from build123d import *

# Parameters (mm, degrees)
F0_W      = 88.9
F0_H      = 228.6
F1_DEPTH  = 19.05
F3_DEPTH  = 19.051
F4_R      = 4.7625
F5_DEPTH  = 5
F6_R      = 2.1
F7_DEPTH  = 12.7
F8_R      = 2.1
F9_DEPTH  = 12.7
F10_R     = 2.1
F10_R_2   = 2.0955
F11_DEPTH = 12.7
F12_W     = 37.5
F12_H     = 142.00124
F13_DEPTH = 0.889
F14_R     = 3.175
F15_DEPTH = 19.051


with BuildPart() as f1:
    # F0 (on Front) → F1 (new body)
    with BuildSketch(Plane.XZ):
        Rectangle(F0_W, F0_H)
    extrude(amount=-F1_DEPTH)

    # F2 (on face) → F3 (cut, through all)
    with BuildSketch(Plane.XZ):
        with BuildLine():
            ThreePointArc((-12.5, 90.3), (-15, 92.8), (-17.5, 90.3))
            Line((-17.5, 90.3), (-12.5, 90.3))
        make_face()
        with BuildLine():
            ThreePointArc((17.5, 90.3), (15, 92.8), (12.5, 90.3))
            Line((12.5, 90.3), (17.5, 90.3))
        make_face()
        with BuildLine():
            Line((17.5, 90.3), (12.5, 90.3))
            ThreePointArc((12.5, 90.3), (15, 87.8), (17.5, 90.3))
        make_face()
        with BuildLine():
            Line((-12.5, 90.3), (-17.5, 90.3))
            ThreePointArc((-17.5, 90.3), (-15, 87.8), (-12.5, 90.3))
        make_face()
        with BuildLine():
            ThreePointArc((-12.5, 60.3), (-15, 62.8), (-17.5, 60.3))
            Line((-17.5, 60.3), (-12.5, 60.3))
        make_face()
        with BuildLine():
            ThreePointArc((17.5, 60.3), (15, 62.8), (12.5, 60.3))
            Line((12.5, 60.3), (17.5, 60.3))
        make_face()
        with BuildLine():
            Line((17.5, 60.3), (12.5, 60.3))
            ThreePointArc((12.5, 60.3), (15, 57.8), (17.5, 60.3))
        make_face()
        with BuildLine():
            Line((-12.5, 60.3), (-17.5, 60.3))
            ThreePointArc((-17.5, 60.3), (-15, 57.8), (-12.5, 60.3))
        make_face()
        with BuildLine():
            ThreePointArc((-12.5, 15.3), (-15, 17.8), (-17.5, 15.3))
            Line((-17.5, 15.3), (-12.5, 15.3))
        make_face()
        with BuildLine():
            ThreePointArc((17.5, 15.3), (15, 17.8), (12.5, 15.3))
            Line((12.5, 15.3), (17.5, 15.3))
        make_face()
        with BuildLine():
            Line((17.5, 15.3), (12.5, 15.3))
            ThreePointArc((12.5, 15.3), (15, 12.8), (17.5, 15.3))
        make_face()
        with BuildLine():
            Line((-12.5, 15.3), (-17.5, 15.3))
            ThreePointArc((-17.5, 15.3), (-15, 12.8), (-12.5, 15.3))
        make_face()
        with BuildLine():
            ThreePointArc((-12.5, -14.7), (-15, -12.2), (-17.5, -14.7))
            Line((-17.5, -14.7), (-12.5, -14.7))
        make_face()
        with BuildLine():
            ThreePointArc((17.5, -14.7), (15, -12.2), (12.5, -14.7))
            Line((12.5, -14.7), (17.5, -14.7))
        make_face()
        with BuildLine():
            Line((17.5, -14.7), (12.5, -14.7))
            ThreePointArc((12.5, -14.7), (15, -17.2), (17.5, -14.7))
        make_face()
        with BuildLine():
            Line((-12.5, -14.7), (-17.5, -14.7))
            ThreePointArc((-17.5, -14.7), (-15, -17.2), (-12.5, -14.7))
        make_face()
    extrude(amount=-F3_DEPTH, mode=Mode.SUBTRACT)

    # F4 (on face) → F5 (cut)
    with BuildSketch(Plane.XZ):
        with Locations((-15, -14.7)):
            Circle(F4_R)
        with Locations((15, -14.7)):
            Circle(F4_R)
        with Locations((15, 15.3)):
            Circle(F4_R)
        with Locations((-15, 15.3)):
            Circle(F4_R)
        with Locations((-15, 60.3)):
            Circle(F4_R)
        with Locations((15, 60.3)):
            Circle(F4_R)
        with Locations((-15, 90.3)):
            Circle(F4_R)
        with Locations((15, 90.3)):
            Circle(F4_R)
    extrude(amount=-F5_DEPTH, mode=Mode.SUBTRACT)

    # F6 (on face) → F7 (cut)
    with BuildSketch(Plane(origin=(-44.45, 0, 0), x_dir=(0, -1, 0), z_dir=(-1, 0, 0))):
        with Locations((-9.525, 88.9)):
            Circle(F6_R)
        with Locations((-9.525, 63.5)):
            Circle(F6_R)
        with Locations((-9.525, 38.1)):
            Circle(F6_R)
        with Locations((-9.525, 12.7)):
            Circle(F6_R)
        with Locations((-9.525, -12.7)):
            Circle(F6_R)
        with Locations((-9.525, -38.1)):
            Circle(F6_R)
        with Locations((-9.525, -63.5)):
            Circle(F6_R)
        with Locations((-9.525, -88.9)):
            Circle(F6_R)
    extrude(amount=-F7_DEPTH, mode=Mode.SUBTRACT)

    # F8 (on face) → F9 (cut)
    with BuildSketch(Plane.YZ.offset(44.45)):
        with Locations((9.525, 88.9)):
            Circle(F8_R)
        with Locations((9.525, 63.5)):
            Circle(F8_R)
        with Locations((9.525, 38.1)):
            Circle(F8_R)
        with Locations((9.525, 12.7)):
            Circle(F8_R)
        with Locations((9.525, -63.5)):
            Circle(F8_R)
        with Locations((9.525, -12.7)):
            Circle(F8_R)
        with Locations((9.525, -38.1)):
            Circle(F8_R)
        with Locations((9.525, -88.9)):
            Circle(F8_R)
    extrude(amount=-F9_DEPTH, mode=Mode.SUBTRACT)

    # F10 (on face) → F11 (cut)
    with BuildSketch(Plane(origin=(0, 0, -114.3), x_dir=(1, 0, 0), z_dir=(0, 0, -1))):
        with Locations((-25.4, -9.525)):
            Circle(F10_R)
        with Locations((25.4, -9.525)):
            Circle(F10_R)
        with Locations((0, -9.525)):
            Circle(F10_R_2)
    extrude(amount=-F11_DEPTH, mode=Mode.SUBTRACT)

    # F12 (on face) → F13 (cut)
    with BuildSketch(Plane(origin=(0, 19.05, 0), x_dir=(-1, 0, 0), z_dir=(0, 1, 0))):
        with Locations((0, 43.29938)):
            Rectangle(F12_W, F12_H)
    extrude(amount=-F13_DEPTH, mode=Mode.SUBTRACT)

    # F14 (on face) → F15 (cut, through all)
    with BuildSketch(Plane.XZ):
        with Locations((-34.925, -50.8)):
            Circle(F14_R)
        with Locations((-34.925, -101.6)):
            Circle(F14_R)
        with Locations((34.925, -50.8)):
            Circle(F14_R)
        with Locations((34.925, -101.6)):
            Circle(F14_R)
    extrude(amount=-F15_DEPTH, mode=Mode.SUBTRACT)


solid = f1.part
Design review of the part built by this model. Coordinates are the model's own, in mm. A direction names the side the tool comes from. Give positions to 0.01 mm unless a question says otherwise; leave off trailing zeros. Write each loop counter-clockwise with the first axis right and the second up, starting at its lowest first coordinate (ties: lowest second). Pieces come first, ordered by that corner, then holes. Notation, with made-up numbers: M -31.5,-28 L 17.5,-28 A16 ccw 17.5,-8 Z; hole C 59.25,-0.75 d11. An arc over 180 degrees is marked long. Answer as a JSON object with one key per item and string values. Group by question number.
1) We need section B-B (z = 82). Give the boundary of the cut face in (x, y).
2) We need section C-C (x = 15). Count the separate pieces of the cut face and the enclosed holes in it, and give its area (3 significant figures).
3) Clearance check with flat-ended pins moving along their axes: pin 1 Ø3.5 at (y, z) = (9.525, 12.7) entering from +X; pin 2 Ø2 at (x, y) = (25, 10.5) entering from -Z; pin 3 Ø5 at (x, z) = (15, 60) entering from -Y. State where each tip first meets the part, or that it passes through.
4) We need section A-A (z = -50.8). Give the boundary of the cut face in (x, y).
5) For line 1 along X through (y, z) = (13, 90.3); line 2 along Z through (x, y) = (15, 1.45); line 3 along X through (y, z) = (9.5, 90.3), list the stretches that pass through material, from the lowest coordinate up.
6) Mouldability with a two-part tool opening along Z and no side actions: class faces 1 (the face through (44.45, 9, -2)), 2 (the face through (-38.19, 9.98, -65.55)) as released by +Z, released by -Z, zero draft, split by the parting line, or undercut.
7) We need section D-D (x = 0). Give the boundary of the cut face in (y, z).
8) Tool access review of faces 3 (the face through (34.24, 9.39, -104.7)), 4 (the face through (-18.78, 2.46, -17.6)), 5 (the face through (31.75, 9, -38)), 6 (the face through (-31.75, 10, -38)): name each direction out of +Z, -Z, +X, -X, +Y, -Y from which nothing blocks a thin tool from reaching the whole face with its end or side.
Answer key:
{
 "1": {"outline": "M -44.45,0 L 44.45,0 L 44.45,19.05 L 18.75,19.05 L 18.75,18.16 L -18.75,18.16 L -18.75,19.05 L -44.45,19.05 Z"},
 "2": {"separate pieces": "5", "enclosed holes": "0", "area": "3,770 mm²"},
 "3": {"pin 1": "stops at x = 31.75", "pin 2": "stops at z = -101.6", "pin 3": "stops at y = 5"},
 "4": {"outline": "M -44.45,0 L -38.1,0 L -38.1,19.05 L -44.45,19.05 Z; M -31.75,0 L 31.75,0 L 31.75,19.05 L -31.75,19.05 Z; M 38.1,0 L 44.45,0 L 44.45,19.05 L 38.1,19.05 Z"},
 "5": {"line 1": "x = -44.45 to -17.5, -12.5 to 12.5, 17.5 to 44.45", "line 2": "z = -114.3 to -19.46, -9.94 to 10.54, 20.06 to 55.54, 65.06 to 85.54, 95.06 to 114.3", "line 3": "x = -31.75 to -17.5, -12.5 to 12.5, 17.5 to 31.75"},
 "6": {"face 1": "zero draft", "face 2": "undercut"},
 "7": {"outline": "M 0,-114.3 L 7.43,-114.3 L 7.43,-101.6 L 11.62,-101.6 L 11.62,-114.3 L 19.05,-114.3 L 19.05,-27.7 L 18.16,-27.7 L 18.16,114.3 L 0,114.3 Z"},
 "8": {"face 3": "+Y, -Y", "face 4": "-Y", "face 5": "+X", "face 6": "-X"}
}
